Work out the finished part from the listing and answer in its coordinate system (mm). Face numbers are marked on the shaded views. A direction names the side the tool comes from. Round coordinates to 2 decimals unless told otherwise and drop trailing zeros. Write each loop counter-clockwise with the first axis right and the second up, starting at its lowest first coordinate (ties: lowest second). Pieces come first, ordered by that corner, then holes. Notation, with made-up numbers: (52, 29) -> (111, 29) arc R34 ccw to (111, 62) -> close; hole circle Ø1 at (10, -14.5). An arc over 180 degrees is marked (long way). One line per item, written item: value.
Solid Edge part; units mm, degrees
sketch "Sketch1" plane through (0, 0, 0) normal (0, -1, 0) x (1, 0, 0)
  line L0 (-21.15, 17.15) -> (-21.15, -17.15)
  line L1 (-21.15, -17.15) -> (-17.15, -21.15)
  line L2 (-17.15, -21.15) -> (17.15, -21.15)
  line L3 (17.15, -21.15) -> (21.15, -17.15)
  line L4 (21.15, -17.15) -> (21.15, 17.15)
  line L5 (21.15, 17.15) -> (17.15, 21.15)
  line L6 (17.15, 21.15) -> (-17.15, 21.15)
  line L7 (-17.15, 21.15) -> (-21.15, 17.15)
  dimension "D1" = 17.15
extrude "Protrusion1" add sketch "Sketch1" along normal mid plane 35
sketch "Sketch2" plane through (0, 0, 0) normal (0, -1, 0) x (1, 0, 0)
  line L0 (-20.15, 16.3391) -> (-20.15, -16.3391)
  line L1 (-20.15, -16.3391) -> (-16.3391, -20.15)
  line L2 (-16.3391, -20.15) -> (16.3391, -20.15)
  line L3 (16.3391, -20.15) -> (20.15, -16.3391)
  line L4 (20.15, -16.3391) -> (20.15, 16.3391)
  line L5 (20.15, 16.3391) -> (16.3391, 20.15)
  line L6 (16.3391, 20.15) -> (-16.3391, 20.15)
  line L7 (-16.3391, 20.15) -> (-20.15, 16.3391)
extrude "ExtrudedCutout_1" cut sketch "Sketch2" along normal mid plane 25 flip side to cut
sketch "Sketch3" plane through (0, 0, 0) normal (1, 0, 0) x (0, 1, 0)
  line L0 (-17.5, 0) -> (-17.5, 11)
  line L1 (-17.5, 11) -> (-19.5, 11)
  line L2 (-19.5, 11) -> (-19.5, 2.5)
  line L3 (-19.5, 2.5) -> (-47.5, 2.5)
  line L4 (-47.5, 2.5) -> (-47.5, 0)
  dimension "D1" = 17.5
revolve "RevolvedProtrusion1" add sketch "Sketch3" angle 360 about axis through (0, -46, 0) along (0, 1, 0)
chamfer "Chamfer_1" distance 0.5 angle 45 2 edges at (0, -19.5, 11) (0, -47.5, 2.5)
hole "Hole_1" at (-15.5, -17.5, -15.5) direction (0, 1, 0) diameter 3.242 depth 4.5 tip angle 118 thread major 4 thread length 4
hole "Hole1" at (-15.5, -17.5, 15.5) direction (0, 1, 0) diameter 3.242 depth 4.5 tip angle 118 thread major 4 thread length 4
hole "Hole2" at (15.5, -17.5, -15.5) direction (0, 1, 0) diameter 3.242 depth 4.5 tip angle 118 thread major 4 thread length 4
hole "Hole3" at (15.5, -17.5, 15.5) direction (0, 1, 0) diameter 3.242 depth 4.5 tip angle 118 thread major 4 thread length 4
properties material "Stainless steel"
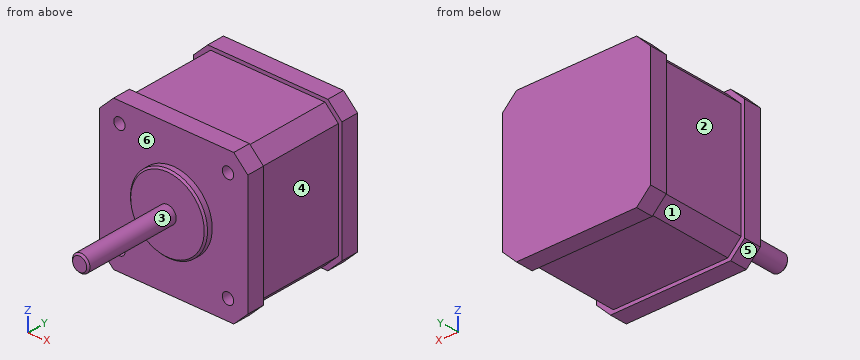
(1) Find section D-D on y = -25. Give the vertices of the cut face in (x, z).
Reported:
outline: circle Ø5 at (0, 0)
(2) Find section A-A on y = -7. Give the vertices of the cut face in (x, z).
Reported:
outline: (-20.15, -16.34) -> (-16.34, -20.15) -> (16.34, -20.15) -> (20.15, -16.34) -> (20.15, 16.34) -> (16.34, 20.15) -> (-16.34, 20.15) -> (-20.15, 16.34) -> close
(3) A tool of negligible diameter and unlimited length cuts with its end or side. For the marked faces 1, 2 and 3, from which of +Z, -Z, +X, -X, +Y, -Y can it reach the whole face along a straight path? Write none if from no direction.
Reported:
face 1: -Z, -X
face 2: +Z, -Z, -X
face 3: -Y
(4) Find section B-B on x = 0. Give the vertices of the cut face in (y, z), plus the area to 3 significant figures.
Reported:
outline: (-47.5, -2) -> (-47, -2.5) -> (-19.5, -2.5) -> (-19.5, -10.5) -> (-19, -11) -> (-17.5, -11) -> (-17.5, -21.15) -> (-12.5, -21.15) -> (-12.5, -20.15) -> (12.5, -20.15) -> (12.5, -21.15) -> (17.5, -21.15) -> (17.5, 21.15) -> (12.5, 21.15) -> (12.5, 20.15) -> (-12.5, 20.15) -> (-12.5, 21.15) -> (-17.5, 21.15) -> (-17.5, 11) -> (-19, 11) -> (-19.5, 10.5) -> (-19.5, 2.5) -> (-47, 2.5) -> (-47.5, 2) -> close
area: 1,610 mm2
(5) Consider probe 1 along Z at (x, y) = (15.5, -15.05); probe 2 along Z at (x, y) = (-15, -15). Determine where each line is inside the solid, lowest interval first.
Reported:
probe 1: z = -21.15 to -17.12, -13.88 to 13.88, 17.12 to 21.15
probe 2: z = -21.15 to -17.04, -13.96 to 13.96, 17.04 to 21.15
(6) For a pull along Y with two mould halves and no side action, classify the marked faces 4, 5 and 6 as pulls with the +Y half, pulls with the -Y half, needs draft (parallel to the pull), parting line crosses it, or undercut.
Reported:
face 4: undercut
face 5: needs draft
face 6: pulls with the -Y half
(7) Find section C-C on x = -13. Give the vertices of the cut face in (y, z).
Reported:
outline: (-17.5, -21.15) -> (-12.5, -21.15) -> (-12.5, -20.15) -> (12.5, -20.15) -> (12.5, -21.15) -> (17.5, -21.15) -> (17.5, 21.15) -> (12.5, 21.15) -> (12.5, 20.15) -> (-12.5, 20.15) -> (-12.5, 21.15) -> (-17.5, 21.15) -> close
(8) Flat-ended cylindrical pins translate along their axes: pin 1 Ø2.5 at (x, z) = (15.5, -15.5) entering from -Y; pin 2 Ø7.5 at (x, y) = (-8, 3.5) entering from +Z; pin 3 Ø4 at (x, y) = (4, -38) entering from -Z; pin 4 Ø10.5 at (x, z) = (-4, 0) entering from -Y. Find the tip coordinate at first contact, or state that the pin passes through.
Reported:
pin 1: stops at y = -12.78
pin 2: stops at z = 20.15
pin 3: stops at z = -1.5
pin 4: stops at y = -47.5
